from build123d import *

# Parameters (mm, degrees)
SKETCH3_R           = 12
SKETCH3_W           = 6.2
SKETCH3_H           = 6.2
BOSS_EXTRUDE1_DEPTH = 5


with BuildPart() as part:
    # Sketch3 → Boss-Extrude1 (new body)
    with BuildSketch(Plane.XY):
        Polygon((-69.296464556, 41.012193309), (-41.012193309, 69.296464556), (-35.355339059, 74.953318806), (35.355339059, 74.953318806), (41.012193309, 69.296464556), (69.296464556, 41.012193309), (79.903066274, 30.405591591), (27.497474683, -22), (-27.497474683, -22), (-79.903066274, 30.405591591), align=None)
        Circle(SKETCH3_R, mode=Mode.SUBTRACT)
        Polygon((-60.599051148, 23.546655814), (-56.214989104, 27.930717857), (-51.830927061, 23.546655814), (-56.214989104, 19.16259377), align=None, mode=Mode.SUBTRACT)
        Polygon((-27.930717857, 56.214989104), (-23.546655814, 60.599051148), (-19.16259377, 56.214989104), (-23.546655814, 51.830927061), align=None, mode=Mode.SUBTRACT)
        Polygon((19.16259377, 56.214989104), (23.546655814, 51.830927061), (27.930717857, 56.214989104), (23.546655814, 60.599051148), align=None, mode=Mode.SUBTRACT)
        with Locations((-23.1, -16.9)):
            Rectangle(SKETCH3_W, SKETCH3_H, mode=Mode.SUBTRACT)
        Polygon((51.830927061, 23.546655814), (56.214989104, 19.16259377), (60.599051148, 23.546655814), (56.214989104, 27.930717857), align=None, mode=Mode.SUBTRACT)
        with Locations((23.1, -16.9)):
            Rectangle(SKETCH3_W, SKETCH3_H, mode=Mode.SUBTRACT)
    extrude(amount=BOSS_EXTRUDE1_DEPTH)


solid = part.part
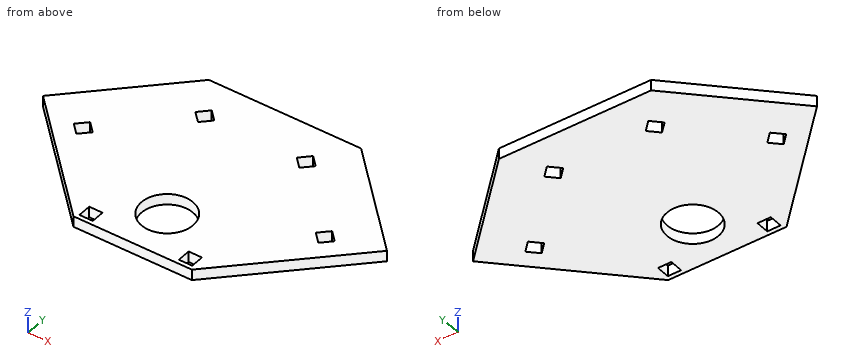
Design review of the part built by this model. Coordinates are the model's own, in mm. Round coordinates to 2 decimals unless told otherwise and drop trailing zeros. Loops run counter-clockwise (first coordinate to the right, second up) from the corner with the lowest first, then second, coordinate; pieces in that order, holes last. Notation, with made-up numbers: (81, 50.25) - (112, 50.25) arc R29 cw to (112, 85.25) - close; hole circle Ø4 at (69, -29.75). An arc over 180 degrees is marked (long way). One line per item, written item: value. Start each with the question number.
1) Consider section A-A on x = 0. Give the boundary of the cut face in (y, z).
2) Consider section B-B on y = 0. Give the boundary of the cut face in (x, z), then the cut area to 3 significant figures.
3) Consider section C-C on x = -21.5. Give the boundary of the cut face in (y, z), then the cut area to 3 significant figures.
4) Consider section D-D on z = 1.9. Give the number of separate pieces and of enclosed holes in the cut face, then the cut area to 3 significant figures.
5) Insertion check: pin 1 Ø1.5 at (y, z) = (-18, 2) entering from -X; pin 2 Ø3 at (y, z) = (49.5, 3.5) entering from +X; pin 3 Ø2 at (y, z) = (38.5, 2.5) entering from +X. Each pin has a flat end and moves straight along its axis. Give the tip position at first contact, or say it passes through.
6) To check wall thickness, follow L1, parallel to Y at x = 0, z = 3.2; L2, parallel to X at y = 24, z = 3.35; L3, parallel to Y at x = -24.5, z = 1.3. State the ranges of each line that lie inside material, in increasing order. Write a range as from..to.
Reported:
1. outline: (-22, 0) - (-12, 0) - (-12, 5) - (-22, 5) - close; (12, 0) - (74.95, 0) - (74.95, 5) - (12, 5) - close
2. outline: (-49.5, 0) - (-12, 0) - (-12, 5) - (-49.5, 5) - close; (12, 0) - (49.5, 0) - (49.5, 5) - (12, 5) - close
2. area: 375 mm^2
3. outline: (-22, 0) - (-20, 0) - (-20, 5) - (-22, 5) - close; (-13.8, 0) - (53.88, 0) - (53.88, 5) - (-13.8, 5) - close; (58.55, 0) - (74.95, 0) - (74.95, 5) - (58.55, 5) - close
3. area: 430 mm^2
4. separate pieces: 1
4. enclosed holes: 7
4. area: 10,100 mm^2
5. pin 1: stops at x = -32.25
5. pin 2: stops at x = 62.31
5. pin 3: stops at x = 72.81
6. L1: y = -22..-12, 12..74.95
6. L2: x = -73.5..-60.15, -52.28..52.28, 60.15..73.5
6. L3: y = -22..-20, -13.8..52.78, 59.65..74.95
